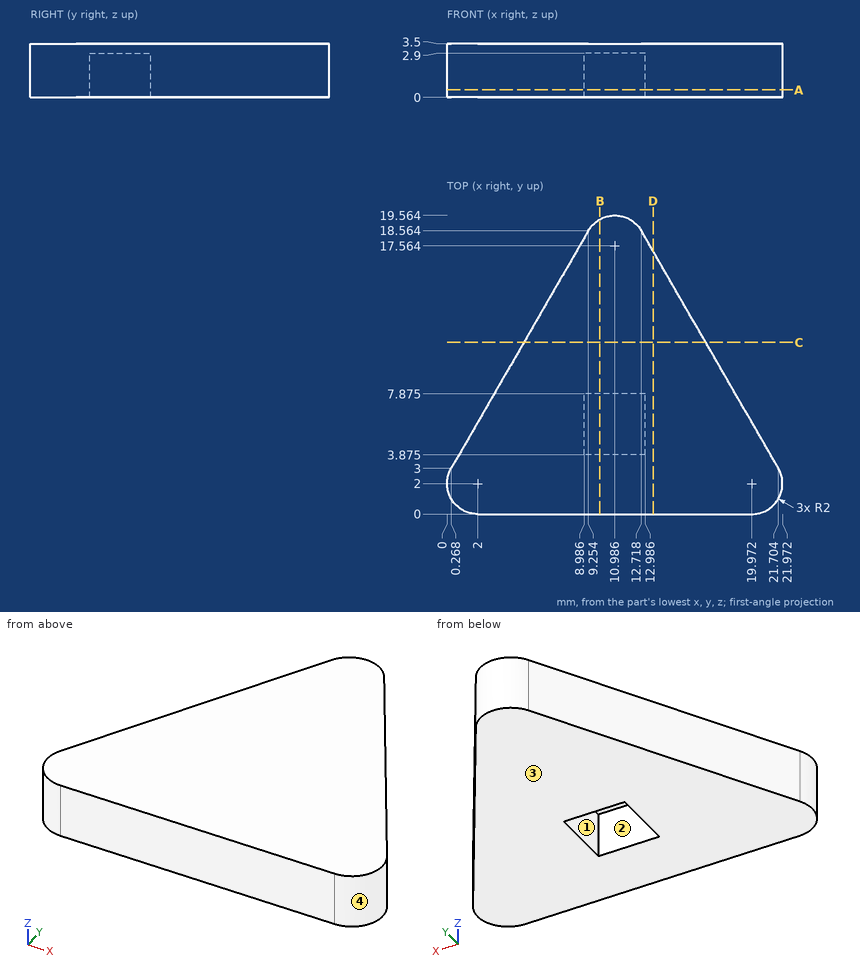
Verification items for this drawing (mm, ordinates from the low corner). Coordinates: 2 decimals unless noted, no trailing zeros. Write each loop counter-clockwise with the first axis right and the second up, starting at its lowest first coordinate (ties: lowest second). Pieces come first, ordered by that corner, then holes. Notation, with made-up numbers: M 64,76 L 105,76 A6 cw 105,81 Z; hole C 38.25,74.5 d8. An arc over 180 degrees is marked long. Answer as CSV lines item,"result".
Q1. Cross-section at C-C (y = 11.25). Record the boundary of the cut face in (x, z).
Check result:
outline,"M 5.03,0 L 16.94,0 L 16.94,3.5 L 5.03,3.5 Z"
Q2. Material ranges on probe 1 along X at (y, z) = (6, 0.7); probe 2 along Z at (x, y) = (12.5, 6.5); probe 3 along Y at (x, z) = (10, 2.55) (1 decimal), recorded low to high. Write a range as from..to.
Check result:
probe 1,"2..8.99, 12.99..19.97"
probe 2,"2.9..3.5"
probe 3,"0..3.9, 7.9..19.3"
Q3. Cross-section at B-B (x = 10). Record the boundary of the cut face in (y, z) (1 decimal).
Check result:
outline,"M 0,0 L 3.9,0 L 3.9,2.9 L 7.9,2.9 L 7.9,0 L 19.3,0 L 19.3,3.5 L 0,3.5 Z"
Q4. Go/stop test with flat-tipped pins: pin 1 (0.9 mm diameter, centred on y = 7, z = 1.5, fed in from +X); pin 2 (2 mm diameter, centred on y = 13.5, z = 2.5, fed in from +X). Record where each tip stops, or that it passes through.
Check result:
pin 1,"x = 19.65"
pin 2,"x = 16.22"
Q5. Cross-section at D-D (x = 13.5). Record the boundary of the cut face in (y, z).
Check result:
outline,"M 0,0 L 17.21,0 L 17.21,3.5 L 0,3.5 Z"
Q6. Mould release check, pull along Y, two halves, no side actions. Record for the marked faces 1, 2, 3 and 4: released by +Y, released by -Y, zero draft, split by the parting line, or undercut.
Check result:
face 1,"undercut"
face 2,"undercut"
face 3,"zero draft"
face 4,"split by the parting line"
Q7. Cross-section at A-A (z = 0.5). Record the boundary of the cut face in (x, y) (1 decimal).
Check result:
outline,"M 0.3,3 A2 ccw 2,0 L 20,0 A2 ccw 21.7,3 L 12.7,18.6 A2 ccw 9.3,18.6 Z; hole M 9,3.9 L 13,3.9 L 13,7.9 L 9,7.9 Z"
